Part model, mm, in its own coordinate system. A direction names the side the tool comes from. Give positions to 0.01 mm unless a question says otherwise; leave off trailing zeros. Write each loop counter-clockwise with the first axis right and the second up, starting at its lowest first coordinate (ties: lowest second). Pieces come first, ordered by that corner, then holes. Notation, with made-up numbers: (-38, -2.75) - (5, -2.75) arc R14 ccw to (5, 14.25) - close; hole circle Ø11 at (51.5, 75.5). An arc over 180 degrees is marked (long way). Answer as a JSON object with one key per item and string values. Group by question number.
```python
from build123d import *

# Parameters (mm, degrees)
SKIZZE1_W                        = 111.8
SKIZZE1_H                        = 38.4
AUFSATZ_LINEAR_AUSTRAGEN1_DEPTH  = 4
SKIZZE2_R                        = 2.4
SCHNITT_LINEAR_AUSTRAGEN1_DEPTH  = 2
LINEARES_MUSTER1_COUNT           = 20
LINEARES_MUSTER1_PITCH           = 8
SKIZZE3_R                        = 2.45
SCHNITT_LINEAR_AUSTRAGEN2_DEPTH  = 69.288871714
SKIZZE3_3_R                      = 3
SKIZZE3_3_R_2                    = 2.45
SCHNITT_LINEAR_AUSTRAGEN3_DEPTH  = 0.9
SKIZZE4_2_R                      = 5
SKIZZE4_2_R_2                    = 1.3
SCHNITT_LINEAR_AUSTRAGEN5_DEPTH  = 69.288871714
SKIZZE4_W                        = 21
SKIZZE4_H                        = 21
SKIZZE4_R                        = 5
SKIZZE4_R_2                      = 1.3
SCHNITT_LINEAR_AUSTRAGEN4_DEPTH  = 2
SKIZZE5_R                        = 4.5
SCHNITT_LINEAR_AUSTRAGEN6_DEPTH  = 69.288871714
SKIZZE5_3_W                      = 41
SKIZZE5_3_H                      = 21
SCHNITT_LINEAR_AUSTRAGEN7_DEPTH  = 7
LOCH_MUSTER_START                = -4
LOCH_MUSTER_OUTLINE_R            = 2.45
LOCH_MUSTER_DEPTH                = 8
LOCH_MUSTER_2_OUTLINE_R          = 3
LOCH_MUSTER_2_OUTLINE_R_2        = 2.45
LOCH_MUSTER_2_DEPTH              = 0.9
LOCH_MUSTER_START_2              = 3.1
LOCH_MUSTER_3_OUTLINE_R          = 3
LOCH_MUSTER_3_OUTLINE_R_2        = 2.45
LOCH_MUSTER_3_DEPTH              = 0.9
FR_SER_10_R                      = 5
FR_SER_4_R                       = 2
M4_GEWINDEBOHRUNG1_D             = 3.3
SCHNITT_LINEAR_AUSTRAGEN8_DEPTH  = 8.5
SKIZZE10_R                       = 2.45
SCHNITT_LINEAR_AUSTRAGEN9_DEPTH  = 16
SKIZZE10_3_R                     = 3
SCHNITT_LINEAR_AUSTRAGEN10_DEPTH = 0.9
M2_GEWINDEBOHRUNG1_D             = 1.6
M2_GEWINDEBOHRUNG1_DEPTH         = 6
M2_GEWINDEBOHRUNG1_TIP           = 0.480688495


# Read off the part's stored shape, not the designer's step: Loch-Muster
with BuildPart() as part:
    # Skizze1 → Aufsatz-Linear austragen1 (new, symmetric)
    with BuildSketch(Plane.XY):
        with Locations((0, 19.2)):
            Rectangle(SKIZZE1_W, SKIZZE1_H)
    extrude(amount=AUFSATZ_LINEAR_AUSTRAGEN1_DEPTH, both=True)

    # Skizze2 → Schnitt-Linear austragen1 (cut)
    with BuildSketch(Plane.XZ):
        with Locations(Location((-52, 0, 0), (0, 0, 270))):
            Circle(SKIZZE2_R)
    schnitt_linear_austragen1 = extrude(amount=-SCHNITT_LINEAR_AUSTRAGEN1_DEPTH, mode=Mode.SUBTRACT)

    # Lineares Muster1: Schnitt-Linear austragen1 ×20
    with Locations(*[(i * LINEARES_MUSTER1_PITCH, 0, 0) for i in range(1, LINEARES_MUSTER1_COUNT)]):
        add(schnitt_linear_austragen1, mode=Mode.SUBTRACT)

    # Skizze3 → Schnitt-Linear austragen2 (cut, through all)
    with BuildSketch(Plane.XY.offset(4)):
        with Locations((0, 8.95)):
            Circle(SKIZZE3_R)
    extrude(amount=-SCHNITT_LINEAR_AUSTRAGEN2_DEPTH, mode=Mode.SUBTRACT)

    # Skizze3<3> → Schnitt-Linear austragen3 (cut)
    with BuildSketch(Plane.XY.offset(4)):
        with Locations((0, 8.95)):
            Circle(SKIZZE3_3_R)
        with Locations((0, 8.95)):
            Circle(SKIZZE3_3_R_2, mode=Mode.SUBTRACT)
    schnitt_linear_austragen3 = extrude(amount=-SCHNITT_LINEAR_AUSTRAGEN3_DEPTH, mode=Mode.SUBTRACT)

    # Spiegeln1: Schnitt-Linear austragen3 across plane
    add(schnitt_linear_austragen3.mirror(Plane.XY), mode=Mode.SUBTRACT)

    # Skizze4<2> → Schnitt-Linear austragen5 (cut, through all)
    with BuildSketch(Plane.XY.offset(4)):
        with Locations((18.998355192, 15.2)):
            Circle(SKIZZE4_2_R)
        with Locations((18.998355192, 23.2)):
            Circle(SKIZZE4_2_R_2)
        with Locations((18.998355192, 7.2)):
            Circle(SKIZZE4_2_R_2)
    extrude(amount=-SCHNITT_LINEAR_AUSTRAGEN5_DEPTH, mode=Mode.SUBTRACT)

    # Skizze4 → Schnitt-Linear austragen4 (cut)
    with BuildSketch(Plane.XY.offset(4)):
        with Locations((18.998355192, 15.2)):
            Rectangle(SKIZZE4_W, SKIZZE4_H)
        with Locations((18.998355192, 15.2)):
            Circle(SKIZZE4_R, mode=Mode.SUBTRACT)
        with Locations((18.998355192, 23.2)):
            Circle(SKIZZE4_R_2, mode=Mode.SUBTRACT)
        with Locations((18.998355192, 7.2)):
            Circle(SKIZZE4_R_2, mode=Mode.SUBTRACT)
    extrude(amount=-SCHNITT_LINEAR_AUSTRAGEN4_DEPTH, mode=Mode.SUBTRACT)

    # Skizze5 → Schnitt-Linear austragen6 (cut, through all)
    with BuildSketch(Plane.XY.offset(4)):
        with Locations((-16, 24.95)):
            Circle(SKIZZE5_R)
    extrude(amount=-SCHNITT_LINEAR_AUSTRAGEN6_DEPTH, mode=Mode.SUBTRACT)

    # Skizze5<3> → Schnitt-Linear austragen7 (cut)
    with BuildSketch(Plane.XY.offset(4)):
        with Locations((-26, 24.95)):
            Rectangle(SKIZZE5_3_W, SKIZZE5_3_H)
    extrude(amount=-SCHNITT_LINEAR_AUSTRAGEN7_DEPTH, mode=Mode.SUBTRACT)

    # Loch-Muster outline → Loch-Muster (cut)
    with BuildSketch(Plane.XY.offset(LOCH_MUSTER_START)):
        with Locations((0, 24.95)):
            Circle(LOCH_MUSTER_OUTLINE_R)
    extrude(amount=LOCH_MUSTER_DEPTH, mode=Mode.SUBTRACT)

    # Loch-Muster 2 outline → Loch-Muster 2 (cut)
    with BuildSketch(Plane.XY.offset(LOCH_MUSTER_START)):
        with Locations((0, 24.95)):
            Circle(LOCH_MUSTER_2_OUTLINE_R)
        with Locations((0, 24.95)):
            Circle(LOCH_MUSTER_2_OUTLINE_R_2, mode=Mode.SUBTRACT)
    extrude(amount=LOCH_MUSTER_2_DEPTH, mode=Mode.SUBTRACT)

    # Loch-Muster 3 outline → Loch-Muster 3 (cut)
    with BuildSketch(Plane.XY.offset(LOCH_MUSTER_START_2)):
        with Locations((0, 24.95)):
            Circle(LOCH_MUSTER_3_OUTLINE_R)
        with Locations((0, 24.95)):
            Circle(LOCH_MUSTER_3_OUTLINE_R_2, mode=Mode.SUBTRACT)
    extrude(amount=LOCH_MUSTER_3_DEPTH, mode=Mode.SUBTRACT)

    # Fräser 10
    fr_ser_10_edges = [part.edges().sort_by_distance(p)[0] for p in [
        (8.498355192, 25.7, 3),
        (29.498355192, 25.7, 3),
        (29.498355192, 4.7, 3),
        (8.498355192, 4.7, 3),
    ]]
    fillet(fr_ser_10_edges, radius=FR_SER_10_R)

    # Fräser 4
    fr_ser_4_edges = [part.edges().sort_by_distance(p)[0] for p in [
        (-46.5, 14.45, 0.5),
        (-46.5, 35.45, 0.5),
        (-5.5, 35.45, 0.5),
        (-5.5, 14.45, 0.5),
    ]]
    fillet(fr_ser_4_edges, radius=FR_SER_4_R)

    # M4 Gewindebohrung1 (through all)
    with Locations(Plane.XY.offset(4)):
        with Locations((-50.25, 29.95), (-50.25, 19.95), (-1.75, 19.95), (-1.75, 29.95)):
            Hole(M4_GEWINDEBOHRUNG1_D / 2)

    # Skizze5<4> → Schnitt-Linear austragen8 (cut)
    with BuildSketch(Plane.XY.offset(4)):
        with BuildLine():
            Line((-18.5, 32.45), (-13.5, 32.45))
            ThreePointArc((-13.5, 32.45), (-9.964466094, 30.985533906), (-8.5, 27.45))
            Line((-8.5, 27.45), (-8.5, 22.45))
            ThreePointArc((-8.5, 22.45), (-9.964466094, 18.914466094), (-13.5, 17.45))
            Line((-13.5, 17.45), (-18.5, 17.45))
            ThreePointArc((-18.5, 17.45), (-22.035533906, 18.914466094), (-23.5, 22.45))
            Line((-23.5, 22.45), (-23.5, 27.45))
            ThreePointArc((-23.5, 27.45), (-22.035533906, 30.985533906), (-18.5, 32.45))
        make_face()
    extrude(amount=-SCHNITT_LINEAR_AUSTRAGEN8_DEPTH, mode=Mode.SUBTRACT)

    # Skizze10 → Schnitt-Linear austragen9 (cut)
    with BuildSketch(Plane(origin=(-55.9, 0, 0), x_dir=(0, 0, -1), z_dir=(1, 0, 0))):
        with Locations(Location((0, 15.35, 0), (0, 0, 180))):
            Circle(SKIZZE10_R)
        with Locations(Location((0, 24.95, 0), (0, 0, 180))):
            Circle(SKIZZE10_R)
    schnitt_linear_austragen9 = extrude(amount=SCHNITT_LINEAR_AUSTRAGEN9_DEPTH, mode=Mode.SUBTRACT)

    # Skizze10<3> → Schnitt-Linear austragen10 (cut)
    with BuildSketch(Plane(origin=(-55.9, 0, 0), x_dir=(0, 0, -1), z_dir=(1, 0, 0))):
        with Locations((0, 15.35)):
            Circle(SKIZZE10_3_R)
        with Locations((0, 24.95)):
            Circle(SKIZZE10_3_R)
    schnitt_linear_austragen10 = extrude(amount=SCHNITT_LINEAR_AUSTRAGEN10_DEPTH, mode=Mode.SUBTRACT)

    # Spiegeln2: Schnitt-Linear austragen9, Schnitt-Linear austragen10 across plane
    add(schnitt_linear_austragen9.mirror(Plane(origin=(0, 0, 0), x_dir=(0, 0, 1), z_dir=(1, 0, 0))), mode=Mode.SUBTRACT)
    add(schnitt_linear_austragen10.mirror(Plane(origin=(0, 0, 0), x_dir=(0, 0, 1), z_dir=(1, 0, 0))), mode=Mode.SUBTRACT)

    # M2 Gewindebohrung1
    with Locations(Plane(origin=(0, 38.4, 0), x_dir=(1, 0, 0), z_dir=(0, 1, 0))):
        with Locations((28.998355192, 0), (8.998355192, 0)):
            Hole(M2_GEWINDEBOHRUNG1_D / 2, depth=M2_GEWINDEBOHRUNG1_DEPTH)
            with Locations((0, 0, -(M2_GEWINDEBOHRUNG1_DEPTH + M2_GEWINDEBOHRUNG1_TIP / 2))):  # 118° drill point
                Cone(0, M2_GEWINDEBOHRUNG1_D / 2, M2_GEWINDEBOHRUNG1_TIP, mode=Mode.SUBTRACT)


solid = part.part
```
1) Drop flat-ended pins along their axis: P1, Ø2.5, axis at y = 24.5, z = 0, coming from the +X side; P2, Ø3, axis at x = -52, z = 0, coming from the -Y side. Give the stop position or say it passes through.
2) Saw through at B-B (y = 34.5). List the corners of the cut face in (x, z).
3) Saw through at C-C (x = -28). List the corners of the cut face in (y, z).
4) Saw through at D-D (x = 12). List the corners of the cut face in (y, z).
5) Saw through at A-A (x = 44). List the corners of the cut face in (y, z), and give its area (3 significant figures).
6) Drill centre lines: line 1 along Y through (x, z) = (0, -3.7); line 2 along Y through (x, z) = (-8.5, 1); line 3 along Y through (x, z) = (20.5, 2.25). Where is each one in solid material? Low to high. Write a range as from..to.
7) Which spindle directions (+Z, -Z, +X, -X, +Y, -Y) get a long thin tool onto all of the face, cutting with end or side? Do faces 5 (the cylindrical face through (-55.456, 27.924, 0.391)), 6 (the flat face through (-31, 25, -3)), 7 (the flat face through (-28, 2, 0)), 8 (the cylindrical face through (-9.93, 18.95, -3.49)). Say none if no direction does.
8) Two-plate mould, pull along Y, no slides. Class faces 1 (the flat face through (-1, 15, -4)), 2 (the flat face through (21, 20, 2)), 3 (the cylindrical face through (28.07, 24.2, 2.99)), 4 (the flat face through (44, 2, 0)): +Y half, -Y half, draft (parallel to the pull), parting line (faces both ways), or undercut.
Checks:
{
 "1": {"P1": "x = 39.9", "P2": "y = 2"},
 "2": {"outline": "(-55.9, -4) - (55.9, -4) - (55.9, 4) - (-5.8, 4) - (-5.8, -3) - (-46.2, -3) - (-46.2, 4) - (-55.9, 4) - close; hole circle Ø1.6 at (9, 0); hole circle Ø1.6 at (29, 0)"},
 "3": {"outline": "(0, -4) - (38.4, -4) - (38.4, 4) - (35.45, 4) - (35.45, -3) - (14.45, -3) - (14.45, 4) - (0, 4) - (0, 2.4) - (2, 2.4) - (2, -2.4) - (0, -2.4) - close"},
 "4": {"outline": "(0, -4) - (38.4, -4) - (38.4, 4) - (25.47, 4) - (25.47, 2) - (4.93, 2) - (4.93, 4) - (0, 4) - (0, 2.4) - (2, 2.4) - (2, -2.4) - (0, -2.4) - close"},
 "5": {"outline": "(0, -4) - (38.4, -4) - (38.4, 4) - (0, 4) - (0, 2.4) - (2, 2.4) - (2, -2.4) - (0, -2.4) - close; hole circle Ø4.9 at (15.35, 0); hole circle Ø4.9 at (24.95, 0)", "area": "260 mm2"},
 "6": {"line 1": "0..5.95, 11.95..21.95, 27.95..38.4", "line 2": "0..14.45, 35.45..38.4", "line 3": "2..4.7, 25.7..38.4"},
 "7": {"face 5": "-X", "face 6": "+Z", "face 7": "-Y", "face 8": "+Z, -Z"},
 "8": {"face 1": "draft", "face 2": "undercut", "face 3": "undercut", "face 4": "-Y half"}
}
